from build123d import *

# Parameters (mm, degrees)
SKETCH1_W           = 101.6
SKETCH1_H           = 50.8
BOSS_EXTRUDE1_DEPTH = 25.4
SKETCH2_W           = 25.4
SKETCH2_H           = 19.05
CUT_EXTRUDE1_DEPTH  = 26.4
SKETCH5_W           = 50.8
SKETCH5_H           = 19.05
BOSS_EXTRUDE3_DEPTH = 38.1
SKETCH7_R           = 6.35
CUT_EXTRUDE2_DEPTH  = 26.4


with BuildPart() as part:
    # Sketch1 → Boss-Extrude1 (new body)
    with BuildSketch(Plane(origin=(0, 0, 0), x_dir=(1, 0, 0), z_dir=(0, 1, 0))):
        with Locations((-7.687438987, 79.657257194)):
            Rectangle(SKETCH1_W, SKETCH1_H)
    extrude(amount=BOSS_EXTRUDE1_DEPTH)

    # Sketch2 → Cut-Extrude1 (cut, through all)
    with BuildSketch(Plane(origin=(0, 25.4, 0), x_dir=(1, 0, 0), z_dir=(0, 1, 0))):
        with Locations((-7.687438987, 95.532257194)):
            Rectangle(SKETCH2_W, SKETCH2_H)
    extrude(amount=-CUT_EXTRUDE1_DEPTH, mode=Mode.SUBTRACT)

    # Sketch5 → Boss-Extrude3 (add)
    with BuildSketch(Plane(origin=(0, 25.4, 0), x_dir=(1, 0, 0), z_dir=(0, 1, 0))):
        with Locations((-7.687438987, 63.782257194)):
            Rectangle(SKETCH5_W, SKETCH5_H)
    extrude(amount=BOSS_EXTRUDE3_DEPTH)

    # Sketch7 → Cut-Extrude2 (cut, through all)
    with BuildSketch(Plane(origin=(0, 25.4, 0), x_dir=(1, 0, 0), z_dir=(0, 1, 0))):
        with Locations((24.062561013, 84.755702101)):
            Circle(SKETCH7_R)
    extrude(amount=-CUT_EXTRUDE2_DEPTH, mode=Mode.SUBTRACT)


solid = part.part
Geometry check sheet. Reference: the model listing, model coordinates, mm. A direction names the side the tool comes from. Give positions to 0.01 mm unless a question says otherwise; leave off trailing zeros. Write each loop counter-clockwise with the first axis right and the second up, starting at its lowest first coordinate (ties: lowest second). Pieces come first, ordered by that corner, then holes.
1) Go/stop test with flat-tipped pins: pin 1 Ø6 at (x, y) = (-4, 29) entering from -Z; pin 2 Ø5.5 at (y, z) = (38.5, -64) entering from -X; pin 3 Ø8 at (y, z) = (31.5, -79) entering from +X; pin 4 Ø12 at (y, z) = (27.5, -63) entering from +X. Record where each tip stops, or that it passes through.
Values follow:
pin 1: stops at z = -73.31
pin 2: stops at x = -33.09
pin 3: passes through
pin 4: stops at x = 43.11
2) Set-up check for faces 4 (the face through (-33.087, 44, -64)), 5 (the face through (17.713, 44, -64)), 6 (the face through (-8, 13, -86.007)): record each of +Z, -Z, +X, -X, +Y, -Y from which the full face is reachable in a straight line by a thin tool's end or side.
Values follow:
face 4: +Z, -Z, -X, +Y
face 5: +Z, -Z, +X, +Y
face 6: -Z, +Y, -Y
3) Cross-section at C-C (z = -60.5). Record the boundary of the cut face in (x, y).
Values follow:
outline: (-58.49, 0) - (43.11, 0) - (43.11, 25.4) - (17.71, 25.4) - (17.71, 63.5) - (-33.09, 63.5) - (-33.09, 25.4) - (-58.49, 25.4) - close
4) Thickness scan on line 1 (X direction, y = 10.5, z = -93); line 2 (X direction, y = 61, z = -72); line 3 (Y direction, x = -5.5, z = -77). Record the ranges inside material, lowest first.
Values follow:
line 1: x = -58.49 to -20.39, 5.01 to 43.11
line 2: x = -33.09 to 17.71
line 3: y = 0 to 25.4
5) Cross-section at D-D (x = 19). Record the boundary of the cut face in (y, z), plus the area to 3 significant figures.
Values follow:
outline: (0, -105.06) - (25.4, -105.06) - (25.4, -88.59) - (0, -88.59) - close; (0, -80.92) - (25.4, -80.92) - (25.4, -54.26) - (0, -54.26) - close
area: 1,100 mm2
6) Release check for a two-part mould opening along X. For faces 1 (the face through (-8, 44, -73.307)), 2 (the face through (43.113, 13, -79)), 3 (the face through (-20.387, 13, -95)) record: released by +X, released by -X, zero draft, split by the parting line, or undercut.
Values follow:
face 1: zero draft
face 2: released by +X
face 3: undercut
7) Cross-section at B-B (y = 17). Record the boundary of the cut face in (x, z).
Values follow:
outline: (-58.49, -105.06) - (-20.39, -105.06) - (-20.39, -86.01) - (5.01, -86.01) - (5.01, -105.06) - (43.11, -105.06) - (43.11, -54.26) - (-58.49, -54.26) - close; hole circle Ø12.7 at (24.06, -84.76)
8) Cross-section at A-A (z = -93.5). Record the boundary of the cut face in (x, y).
Values follow:
outline: (-58.49, 0) - (-20.39, 0) - (-20.39, 25.4) - (-58.49, 25.4) - close; (5.01, 0) - (43.11, 0) - (43.11, 25.4) - (5.01, 25.4) - close
